Check sheet for the drawn part. Datum: minimum x, y, z corner. Units: mm. A direction names the side the tool comes from. Round coordinates to 2 decimals unless told otherwise and drop trailing zeros. Write each loop counter-clockwise with the first axis right and the second up, starting at its lowest first coordinate (ties: lowest second). Pieces come first, ordered by that corner, then holes. Notation, with made-up numbers: M 42,-33 L 82,-33 A15 ccw 82,-19 Z; hole C -29.75,-36 d3. An arc over 180 degrees is marked long. One line per item, written item: value.
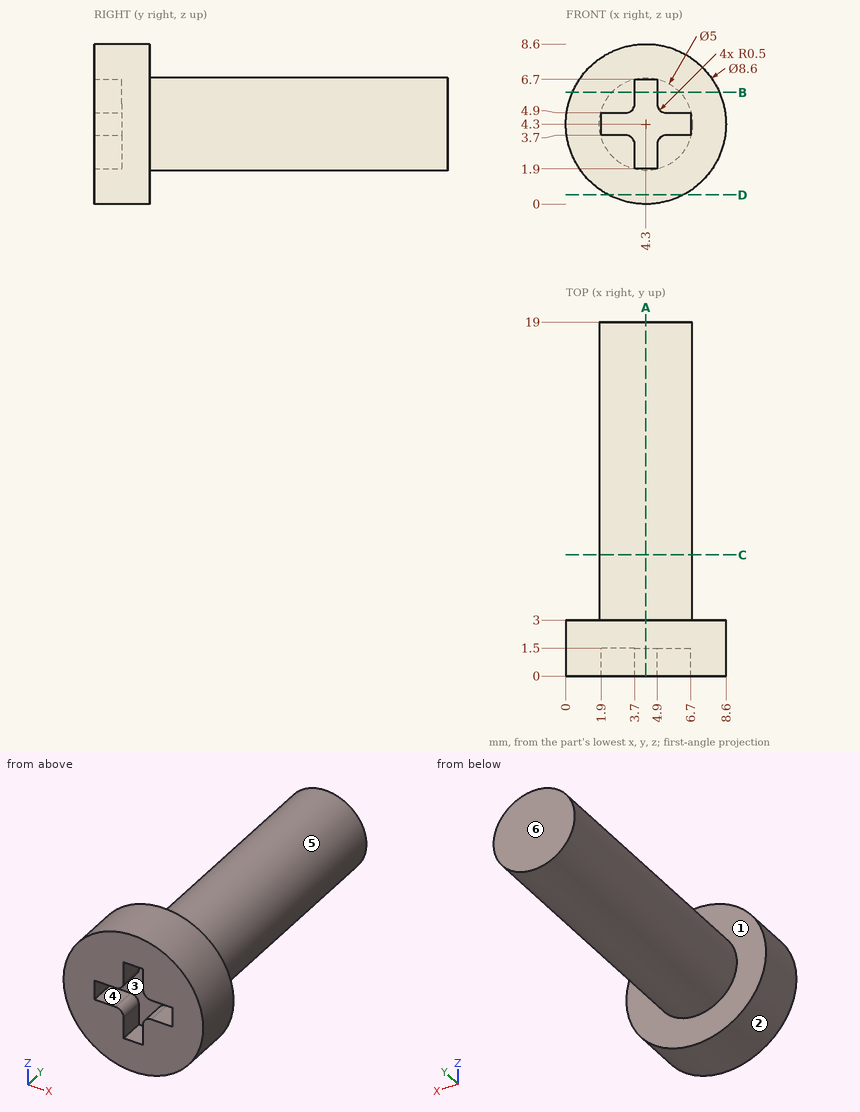
Q1. Scan lines: line 1 (Y direction, x = 5.25, z = 7); line 2 (X direction, y = 12.75, z = 3.25); line 3 (X direction, y = 17.25, z = 5.75). Record each from-to range of solid material in increasing order. Write a range as [from, to].
Completed:
line 1: [0, 3]
line 2: [2.03, 6.57]
line 3: [2.26, 6.34]
Q2. Sectioned sample at D-D on z = 0.5. Enter the section's corners in (x, y).
Completed:
outline: M 2.29,0 L 6.31,0 L 6.31,3 L 2.29,3 Z
Q3. Depth check by flat-ended pin: P1, Ø1.5, axis at y = 15.5, z = 6, coming from the -X side; P2, Ø1.4, axis at x = 6.5, y = 1, coming from the -Z side; P3, Ø0.6, axis at x = 2.5, y = 0.5, coming from the +Z side. Enter the tip coordinate at first touch or a pass-through.
Completed:
P1: x = 1.99
P2: z = 0.27
P3: z = 8.33
Q4. Sectioned sample at A-A on x = 4.3. Enter the section's corners in (y, z).
Completed:
outline: M 0,0 L 3,0 L 3,1.8 L 19,1.8 L 19,6.8 L 3,6.8 L 3,8.6 L 0,8.6 L 0,6.7 L 1.5,6.7 L 1.5,1.9 L 0,1.9 Z
Q5. Sectioned sample at B-B on z = 6. Enter the section's corners in (x, y), and give its area (3 significant figures).
Completed:
outline: M 0.35,0 L 3.7,0 L 3.7,1.5 L 4.9,1.5 L 4.9,0 L 8.25,0 L 8.25,3 L 6.13,3 L 6.13,19 L 2.47,19 L 2.47,3 L 0.35,3 Z
area: 80.6 mm^2
Q6. Access from +Z, -Z, +X, -X, +Y, -Y to the whole of each face (thin tool, end or side, straight path). Record for the marked faces 4, 5 and 6.
Completed:
face 4: -Y
face 5: +Y
face 6: +Z, -Z, +X, -X, +Y
Q7. Sectioned sample at C-C on y = 6.5. Enter the section's corners in (x, z), and give its area (3 significant figures).
Completed:
outline: C 4.3,4.3 d5
area: 19.6 mm^2
Q8. Draft check along Z on the marked faces 1, 2 and 3. Enter one of: pulls with the +Z half, pulls with the -Z half, needs draft (parallel to the pull), parting line crosses it, or undercut.
Completed:
face 1: needs draft
face 2: parting line crosses it
face 3: undercut
